from build123d import *

# Parameters (mm, degrees)
SKETCH1_R           = 1.1303
SKETCH1_R_2         = 1.4732
BOSS_EXTRUDE1_DEPTH = 1.27
FILLET1_R           = 1.5875


with BuildPart() as part:
    # Sketch1 → Boss-Extrude1 (new body)
    with BuildSketch(Plane.XY):
        Polygon((23, 0), (0, 0), (0, -30), (23, -30), (23, -25), (24, -25), (24, -30), (56, -30), (56, -25), (57, -25), (57, -30), (80, -30), (80, 0), (57, 0), (57, -5), (56, -5), (56, 0), (24, 0), (24, -5), (23, -5), align=None)
        with Locations((7, -26.225)):
            Circle(SKETCH1_R, mode=Mode.SUBTRACT)
        with Locations((18, -26.225)):
            Circle(SKETCH1_R, mode=Mode.SUBTRACT)
        with Locations((29, -26.225)):
            Circle(SKETCH1_R, mode=Mode.SUBTRACT)
        with Locations((40, -26.225)):
            Circle(SKETCH1_R, mode=Mode.SUBTRACT)
        with Locations((51, -26.225)):
            Circle(SKETCH1_R, mode=Mode.SUBTRACT)
        with Locations((62, -26.225)):
            Circle(SKETCH1_R, mode=Mode.SUBTRACT)
        with Locations((73, -26.225)):
            Circle(SKETCH1_R, mode=Mode.SUBTRACT)
        with Locations((7, -11.525)):
            Circle(SKETCH1_R, mode=Mode.SUBTRACT)
        with Locations((18, -11.525)):
            Circle(SKETCH1_R, mode=Mode.SUBTRACT)
        with Locations((31, -10)):
            Circle(SKETCH1_R_2, mode=Mode.SUBTRACT)
        with Locations((40, -11.525)):
            Circle(SKETCH1_R, mode=Mode.SUBTRACT)
        with Locations((49, -10)):
            Circle(SKETCH1_R_2, mode=Mode.SUBTRACT)
        with Locations((62, -11.525)):
            Circle(SKETCH1_R, mode=Mode.SUBTRACT)
        with Locations((73, -11.525)):
            Circle(SKETCH1_R, mode=Mode.SUBTRACT)
    extrude(amount=BOSS_EXTRUDE1_DEPTH)

    # Fillet1
    fillet1_edges = [part.edges().sort_by_distance(p)[0] for p in [
        (0, -30, 0.635),
        (0, 0, 0.635),
        (80, 0, 0.635),
        (80, -30, 0.635),
    ]]
    fillet(fillet1_edges, radius=FILLET1_R)


solid = part.part
Here's how the part is built. I have some questions about the finished solid (model axes, mm). Round coordinates to 2 decimals unless told otherwise and drop trailing zeros. Loops run counter-clockwise (first coordinate to the right, second up) from the corner with the lowest first, then second, coordinate; pieces in that order, holes last. Notation, with made-up numbers: (40.5, 60.25) - (61.5, 60.25) arc R32 cw to (61.5, 86.25) - close; hole circle Ø1 at (78, 84). An arc over 180 degrees is marked (long way). One line per question, with ' | ' between items. Start each with the question number.
Q1. Please list where these lines run through material, in increasing order: line 1 (X direction, y = -4.25, z = 0.5); line 2 (Y direction, x = 18, z = 0.6); line 3 (Y direction, x = 31, z = 0.95). Write a range as [from, to].
Q2. I want a section at B-B (z = 0.95). State how many separate pieces and enclosed holes the cut face has, then the cut area to 3 significant figures.
Q3. We'd pull the mould along Y, two halves only. Please class faces 1 (the cylindrical face through (0.45, -29.52, 0.64)), 2 (the flat face through (39, -15, 1.27)), 3 (the cylindrical face through (8, -11, 1)): +Y half, -Y half, draft (parallel to the pull), parting line (faces both ways), or undercut.
Q4. Will this pin go through, and if not, where does the flat tip stop? pin 1 (1.4 mm diameter, centred on x = 18, y = -11.525, fed in from +Z).
Q5. I want a section at A-A (x = 7). Write out the boundary of the cut face in (y, z).
Response values:
1) line 1: x = [0, 23], [24, 56], [57, 80] | line 2: y = [-30, -27.36], [-25.09, -12.66], [-10.39, 0] | line 3: y = [-30, -11.47], [-8.53, 0]
2) separate pieces: 1 | enclosed holes: 14 | area: 2,320 mm²
3) face 1: -Y half | face 2: draft | face 3: undercut
4) pin 1: passes through
5) outline: (-30, 0) - (-27.36, 0) - (-27.36, 1.27) - (-30, 1.27) - close; (-25.09, 0) - (-12.66, 0) - (-12.66, 1.27) - (-25.09, 1.27) - close; (-10.39, 0) - (0, 0) - (0, 1.27) - (-10.39, 1.27) - close
